Autodesk Inventor part; units mm, degrees
ref_plane "YZ Plane" through (0, 0, 0) normal (1, 0, 0) x (0, 1, 0)
ref_plane "XZ Plane" through (0, 0, 0) normal (0, 1, 0) x (-1, 0, 0)
ref_plane "XY Plane" through (0, 0, 0) normal (0, 0, 1) x (1, 0, 0)
sketch "Sketch1" plane through (0, 0, 0) normal (0, 0, 1) x (1, 0, 0)
  circle A0 centre (0, 0) radius 15
  dimension "d0" = 30
extrude "Extrusion1" add sketch "Sketch1" along normal blind 8
sketch "Sketch2" plane through (0, 0, 8) normal (0, 0, 1) x (1, 0, 0)
  circle A0 centre (0, 0) radius 15
  line L0 (-3.7816, 6.55) -> (0, 6.55)
  line L1 (3.7816, 6.55) -> (7.5633, 0)
  line L2 (7.5633, 0) -> (3.7816, -6.55)
  line L3 (3.7816, -6.55) -> (-3.7816, -6.55)
  line L4 (-3.7816, -6.55) -> (-7.5633, 0)
  line L5 (-7.5633, 0) -> (-3.7816, 6.55)
  line L6 (0, -15) -> (0, -6.55)
  line L7 (-15, 0) -> (-7.5633, 0)
  line L8 (0, 6.55) -> (0, 15)
  line L9 (7.5633, 0) -> (15, 0)
  line L10 (0, 6.55) -> (3.7816, 6.55)
  dimension "d4" = 13.1
extrude "Extrusion2" add sketch "Sketch2" along normal blind 4 contours A0 L6 L3 L2 L9 | L8 L0 L5 L7 A0
sketch "Sketch3" plane through (0, 0, 8) normal (0, 0, 1) x (1, 0, 0)
  arc A0 (-15, 0) -> (0, -15) centre (0, 0) ccw
  line L0 (-3.7816, 6.55) -> (3.7816, 6.55)
  line L1 (3.7816, 6.55) -> (7.5633, 0)
  line L2 (7.5633, 0) -> (3.7816, -6.55)
  line L3 (3.7816, -6.55) -> (-3.7816, -6.55)
  line L4 (-3.7816, -6.55) -> (-7.5633, 0)
  line L5 (-7.5633, 0) -> (-3.7816, 6.55)
extrude "Extrusion3" cut sketch "Sketch3" against normal blind 4
sketch "Sketch4" plane through (0, 0, 4) normal (0, 0, 1) x (1, 0, 0)
  circle A0 centre (0, 0) radius 3.9
  dimension "d10" = 7.8
extrude "Extrusion4" cut sketch "Sketch4" against normal blind 10
properties part number "Coil Coupling_1"
Work out the finished part from the listing and answer in its coordinate system (mm). A direction names the side the tool comes from. Give positions to 0.01 mm unless a question says otherwise; leave off trailing zeros. Loops run counter-clockwise (first coordinate to the right, second up) from the corner with the lowest first, then second, coordinate; pieces in that order, holes last. Notation, with made-up numbers: (20, 30) -> (41, 30) arc R20 cw to (41, 36) -> close; hole circle Ø2 at (21.25, 21.25). An arc over 180 degrees is marked (long way). Use a Markdown table: item, result. Add a question column.
1) The part is cut by section C-C, the plane x = 9.75. Determine the outline of the cut face in (y, z).
2) The part is cut by section B-B, the plane y = -1.5. Determine the outline of the cut face in (x, z).
3) Each of these flat-tipped pins is pushed along its axis until it touches: P1, Ø4, axis at x = -2, z = 8, coming from the -Y side; P2, Ø5, axis at y = -3.5, z = 7, coming from the -X side; P3, Ø1.5, axis at x = -11.5, z = 10.5, coming from the +Y side; P4, Ø2, axis at y = -9, z = 9.5, coming from the -X side. Where does it stop, or does it pass through?
4) Consider line 1 along Y through (x, z) = (0, 1.1); line 2 along Z through (x, y) = (-0.5, -6); line 3 along Z through (x, y) = (-7.5, -12.5). Determine where each line is inside the solid, lowest interval first.
5) For a pull along Y with two mould halves and no side action, classify faces 1 (the flat face through (11, 0, 10)), 2 (the flat face through (3, -3, 0)), 3 (the flat face through (-5.646, -3.321, 6.028)), 4 (the flat face through (-5.7, 3.23, 7.94)) as +Y half, -Y half, draft (parallel to the pull), parting line (faces both ways), or undercut.
6) Which of the six approach directions +Z, -Z, +X, -X, +Y, -Y give full straight-line access (tool end or side, diameter ignored) to faces 5 (the flat face through (7, 8, 8)), 6 (the flat face through (-11, 0, 10)), 7 (the flat face through (1, -6.55, 7))?
7) The part is cut by section A-A, the plane z = 7. Determine the outline of the cut face in (x, y).
8) The part is cut by section D-D, the plane y = -9. Determine the outline of the cut face in (x, z).
Reported:
| question | item | result |
|---|---|---|
| 1 | outline | (-11.4, 0) -> (11.4, 0) -> (11.4, 8) -> (0, 8) -> (0, 12) -> (-11.4, 12) -> close |
| 2 | outline | (-14.92, 0) -> (-3.6, 0) -> (-3.6, 4) -> (-6.7, 4) -> (-6.7, 8) -> (-14.92, 8) -> close; (3.6, 0) -> (14.92, 0) -> (14.92, 12) -> (6.7, 12) -> (6.7, 4) -> (3.6, 4) -> close |
| 3 | P1 | stops at y = -15 |
| 3 | P2 | stops at x = -14.97 |
| 3 | P3 | stops at y = 10.46 |
| 3 | P4 | stops at x = 0 |
| 4 | line 1 | y = -15 to -3.9, 3.9 to 15 |
| 4 | line 2 | z = 0 to 4 |
| 4 | line 3 | z = 0 to 8 |
| 5 | face 1 | +Y half |
| 5 | face 2 | draft |
| 5 | face 3 | undercut |
| 5 | face 4 | undercut |
| 6 | face 5 | +Z, +X, +Y |
| 6 | face 6 | +Z, -X, -Y |
| 6 | face 7 | +Z |
| 7 | outline | circle Ø30 at (0, 0); hole (-7.56, 0) -> (-3.78, -6.55) -> (3.78, -6.55) -> (7.56, 0) -> (3.78, 6.55) -> (-3.78, 6.55) -> close |
| 8 | outline | (-12, 0) -> (12, 0) -> (12, 12) -> (0, 12) -> (0, 8) -> (-12, 8) -> close |
